```python
from build123d import *

# Parameters (mm, degrees)
BOSS_EXTRUDE1_DEPTH = 25
SKETCH2_R           = 1
SKETCH2_R_2         = 6
CUT_EXTRUDE1_DEPTH  = 53
FILLET2_R           = 2
SKETCH3_R           = 1.5
CUT_EXTRUDE2_DEPTH  = 42


with BuildPart() as part:
    # Sketch1 → Boss-Extrude1 (new body)
    with BuildSketch(Plane(origin=(0, 0, 0), x_dir=(1, 0, 0), z_dir=(0, 1, 0))):
        Polygon((-21.5, 0.5), (28.5, 0.5), (28.5, 40.5), (29.5, 40.5), (29.5, 0.5), (29.5, -0.5), (-22.5, -0.5), (-22.5, 0.5), (-22.5, 40.5), (-21.5, 40.5), align=None)
    extrude(amount=BOSS_EXTRUDE1_DEPTH)

    # Sketch2 → Cut-Extrude1 (cut, through all)
    with BuildSketch(Plane(origin=(29.5, 0, 0), x_dir=(0, 0, -1), z_dir=(1, 0, 0))):
        with Locations((28.5, 12.5)):
            Circle(SKETCH2_R)
        with Locations((38, 12.5)):
            Circle(SKETCH2_R_2)
        with Locations((31.282485579, 19.217514421)):
            Circle(SKETCH2_R)
        with Locations((38, 22)):
            Circle(SKETCH2_R)
        with Locations((38, 3)):
            Circle(SKETCH2_R)
        with Locations((31.282485579, 5.782485579)):
            Circle(SKETCH2_R)
    extrude(amount=-CUT_EXTRUDE1_DEPTH, mode=Mode.SUBTRACT)

    # Fillet2
    fillet2_edges = [part.edges().sort_by_distance(p)[0] for p in [
        (29.5, 12.5, 0.5),
        (-22.5, 12.5, 0.5),
        (-21.5, 12.5, -0.5),
        (28.5, 12.5, -0.5),
    ]]
    fillet(fillet2_edges, radius=FILLET2_R)

    # Sketch3 → Cut-Extrude2 (cut, through all)
    with BuildSketch(Plane.XY.offset(0.5)):
        with Locations((-13.5, 20)):
            Circle(SKETCH3_R)
        with Locations((20.5, 20)):
            Circle(SKETCH3_R)
        with Locations((-13.5, 5)):
            Circle(SKETCH3_R)
        with Locations((20.5, 5)):
            Circle(SKETCH3_R)
    extrude(amount=-CUT_EXTRUDE2_DEPTH, mode=Mode.SUBTRACT)


solid = part.part
```
Geometry: final body of the model. Coordinates: model frame, mm. A direction names the side the tool comes from. Coordinates: 2 decimals unless noted, no trailing zeros. Order: outer loops, then holes, each group sorted by start corner. A loop starts at its lowest first (then second) coordinate and runs counter-clockwise, first axis right, second up.
Item 1: Section query A-A (z = -26.5). Output: boundary loops of the cut face in (x, y).
Answer:
outline: (-22.5, 0) - (-21.5, 0) - (-21.5, 25) - (-22.5, 25) - close; (28.5, 0) - (29.5, 0) - (29.5, 25) - (28.5, 25) - close
Item 2: Draft query along X for faces 1 (the face through (-21.5, 12, -22)), 2 (the face through (-21.9, 12.68, -0.07)), 3 (the face through (29, 3, -39)). Return one class per face: released by +X, released by -X, zero draft, split by the parting line, or undercut.
Answer:
face 1: undercut
face 2: released by -X
face 3: zero draft
Item 3: Section query D-D (y = 9.25). Output: boundary loops of the cut face in (x, z), then the cut area to 3 significant figures.
Answer:
outline: (-22.5, -32.96) - (-21.5, -32.96) - (-21.5, -2.5) arc R2 cw to (-19.5, -0.5) - (26.5, -0.5) arc R2 cw to (28.5, -2.5) - (28.5, -32.96) - (29.5, -32.96) - (29.5, -1.5) arc R2 ccw to (27.5, 0.5) - (-20.5, 0.5) arc R2 ccw to (-22.5, -1.5) - close
area: 117 mm2
Item 4: Section query B-B (x = -13.5). Output: boundary loops of the cut face in (y, z).
Answer:
outline: (0, -0.5) - (3.5, -0.5) - (3.5, 0.5) - (0, 0.5) - close; (6.5, -0.5) - (18.5, -0.5) - (18.5, 0.5) - (6.5, 0.5) - close; (21.5, -0.5) - (25, -0.5) - (25, 0.5) - (21.5, 0.5) - close
Item 5: Access query for faces 4 (the face through (27.9, 12.68, -1.07)), 5 (the face through (19, 5, 0)). Directions: +Z, -Z, +X, -X, +Y, -Y. A direction counts if a zero-diameter tool reaches every point of the face in a straight line with its end or side. Return the directions, or none.
Answer:
face 4: -Z, +Y, -Y
face 5: +Z, -Z
Item 6: Section query C-C (y = 12.5). Output: boundary loops of the cut face in (x, z).
Answer:
outline: (-22.5, -32) - (-21.5, -32) - (-21.5, -29.5) - (-22.5, -29.5) - close; (-22.5, -27.5) - (-21.5, -27.5) - (-21.5, -2.5) arc R2 cw to (-19.5, -0.5) - (26.5, -0.5) arc R2 cw to (28.5, -2.5) - (28.5, -27.5) - (29.5, -27.5) - (29.5, -1.5) arc R2 ccw to (27.5, 0.5) - (-20.5, 0.5) arc R2 ccw to (-22.5, -1.5) - close; (28.5, -32) - (29.5, -32) - (29.5, -29.5) - (28.5, -29.5) - close
Item 7: Material intervals for line 1 along X through (y, z) = (1.25, -32.5); line 2 along Y through (x, z) = (-21.95, -38); line 3 along Z through (x, y) = (0, 17), sorted ascending.
Answer:
line 1: x = -22.5 to -21.5, 28.5 to 29.5
line 2: y = 0 to 2, 4 to 6.5, 18.5 to 21, 23 to 25
line 3: z = -0.5 to 0.5
Item 8: Contact query for a flat-ended pin moving along its axis: P1, Ø12, axis at x = 11.5, y = 2.5, coming from the -Z side. Output: stop coordinate, or through.
Answer:
P1: stops at z = -0.5
